```python
from build123d import *

# Parameters (mm, degrees)
SKETCH001_W   = 180
SKETCH001_H   = 60
SKETCH001_W_2 = 15
SKETCH001_H_2 = 3
SKETCH001_W_3 = 3
SKETCH001_H_3 = 15
PAD_DEPTH     = 2
SKETCH_R      = 7.5
SKETCH_W      = 12
SKETCH_H      = 6
POCKET_DEPTH  = 2


with BuildPart() as part:
    # Sketch001 → Pad (new body)
    with BuildSketch(Plane.XY):
        with Locations((90, 30)):
            Rectangle(SKETCH001_W, SKETCH001_H)
        with Locations((36.5, 61.5)):
            Rectangle(SKETCH001_W_2, SKETCH001_H_2)
        with Locations((36.5, -1.5)):
            Rectangle(SKETCH001_W_2, SKETCH001_H_2)
        with Locations((143.5, 61.5)):
            Rectangle(SKETCH001_W_2, SKETCH001_H_2)
        with Locations((143.5, -1.5)):
            Rectangle(SKETCH001_W_2, SKETCH001_H_2)
        with Locations((-1.5, 30)):
            Rectangle(SKETCH001_W_3, SKETCH001_H_3)
        with Locations((181.5, 30)):
            Rectangle(SKETCH001_W_3, SKETCH001_H_3)
    extrude(amount=PAD_DEPTH)

    # Sketch → Pocket (cut)
    with BuildSketch(Plane.XY):
        with Locations((36.5, 30)):
            Circle(SKETCH_R)
        with Locations((143.5, 30)):
            Circle(SKETCH_R)
        with Locations((96, 8)):
            Rectangle(SKETCH_W, SKETCH_H)
    extrude(amount=POCKET_DEPTH, mode=Mode.SUBTRACT)


solid = part.part
```
Here's how the part is built. I have some questions about the finished solid (model axes, mm). Coordinates: 2 decimals unless noted, no trailing zeros. Order: outer loops, then holes, each group sorted by start corner. A loop starts at its lowest first (then second) coordinate and runs counter-clockwise, first axis right, second up. Notation, with made-up numbers: M 26.25,86.25 L 30.25,86.25 A30 ccw 30.25,119.25 Z; hole C 46,74 d7. An arc over 180 degrees is marked long. Answer as a JSON object with one key per item and string values. Group by question number.
(1) I need wall thicknesses on probe 1 along Y at (x, z) = (143.5, 0.75); probe 2 along X at (y, z) = (25, 0.4); probe 3 along X at (y, z) = (18, 1.4). Which ranges of each line are inside material? Lowest first, please.
(2) If we mould it in two halves opening along X, with no side actions, what happens to faces 1 (the face through (150.43, 27.13, 0.99)), 2 (the face through (89, 30, 0)), 3 (the face through (34.87, 22.68, 0.99))? For each: released by +X, released by -X, zero draft, split by the parting line, or undercut.
(3) Suppose I cut it at A-A, the plane y = 30. Please give me the cut outline in (x, z).
(4) Suppose I cut it at D-D, the plane y = 56. Please give me the cut outline in (x, z).
(5) For pin 1 (1 mm diameter, centred on y = -2, z = 1, fed in from -X); pin 2 (0.6 mm diameter, centred on x = 16.5, z = 1.5, fed in from +Y); pin 3 (0.6 mm diameter, centred on y = 43.5, z = 1, fed in from -X), each with a flat end and sliding along its axis, tell me the tip position at first contact or that it passes through.
(6) Suppose I cut it at B-B, the plane x = 143.5. Please give me the cut outline in (y, z).
(7) Suppose I cut it at C-C, the plane z = 1.35. State how many separate pieces and enclosed holes the cut face has, then the cut area to 3 significant figures.
Values found:
{
 "1": {"probe 1": "y = -3 to 22.5, 37.5 to 63", "probe 2": "x = -3 to 30.91, 42.09 to 137.91, 149.09 to 183", "probe 3": "x = 0 to 180"},
 "2": {"face 1": "undercut", "face 2": "zero draft", "face 3": "undercut"},
 "3": {"outline": "M -3,0 L 29,0 L 29,2 L -3,2 Z; M 44,0 L 136,0 L 136,2 L 44,2 Z; M 151,0 L 183,0 L 183,2 L 151,2 Z"},
 "4": {"outline": "M 0,0 L 180,0 L 180,2 L 0,2 Z"},
 "5": {"pin 1": "stops at x = 29", "pin 2": "stops at y = 60", "pin 3": "stops at x = 0"},
 "6": {"outline": "M -3,0 L 22.5,0 L 22.5,2 L -3,2 Z; M 37.5,0 L 63,0 L 63,2 L 37.5,2 Z"},
 "7": {"separate pieces": "1", "enclosed holes": "3", "area": "10,600 mm^2"}
}
